For this review, take the finished solid that the model builds, in its own axes (mm). Round coordinates to 2 decimals unless told otherwise and drop trailing zeros. Write each loop counter-clockwise with the first axis right and the second up, starting at its lowest first coordinate (ties: lowest second). Pieces come first, ordered by that corner, then holes. Notation, with made-up numbers: (-39, 79.5) -> (5, 79.5) arc R10 cw to (5, 87.5) -> close; hole circle Ø7 at (-31.5, 41). An arc over 180 degrees is marked (long way). Write each question's results on one line, items separated by ' | '. Start each with the question number.
Item 1: Add section C-C (x = 86.5). State the section outline as (y, z) points.
Item 2: Add section B-B (y = 86.5). State the section outline as (x, z) points.
Item 3: Add section A-A (z = 2.25). State the section outline as (x, y) points.
Item 4: Clearance check with a flat-ended pin moving along its axis: pin 1 (3 mm diameter, centred on y = 55, z = 4.5, fed in from +X). State where the tip first meets the part, or that it passes through.
Item 5: To check wall thickness, follow line 1 along X through (y, z) = (71, 3.5); line 2 along X through (y, z) = (549.5, 2.5). State the ranges of each line that lie inside material, in increasing order.
from build123d import *

# Parameters (mm, degrees)
F1_DEPTH = 6.35


with BuildPart() as f1:
    # F0 (on Top) → F1 (new body)
    with BuildSketch(Plane.XY):
        Polygon((0, 152.4), (0, 0), (76.2, 0), (76.2, 152.4), (76.2, 585.159104), (0, 585.159104), align=None)
        Polygon((76.2, 585.159104), (76.2, 152.4), (146.001304, 585.159104), align=None)
    extrude(amount=F1_DEPTH)


solid = f1.part
Responses:
1) outline: (216.26, 0) -> (585.16, 0) -> (585.16, 6.35) -> (216.26, 6.35) -> close
2) outline: (0, 0) -> (76.2, 0) -> (76.2, 6.35) -> (0, 6.35) -> close
3) outline: (0, 0) -> (76.2, 0) -> (76.2, 152.4) -> (146, 585.16) -> (0, 585.16) -> close
4) pin 1: stops at x = 76.2
5) line 1: x = 0 to 76.2 | line 2: x = 0 to 140.25
